Source: CAD feature listing. Evaluate the final solid. Frame: model axes, mm. A direction names the side the tool comes from. Round coordinates to 2 decimals unless told otherwise and drop trailing zeros. Loops run counter-clockwise (first coordinate to the right, second up) from the corner with the lowest first, then second, coordinate; pieces in that order, holes last. Notation, with made-up numbers: (-3, 16) -> (55, 16) arc R25 ccw to (55, 35) -> close; hole circle Ø7 at (-13.75, 45.25). An arc over 180 degrees is marked (long way). Write item = value, one per line.
from build123d import *

# Parameters (mm, degrees)
PAD_DEPTH      = 4
PAD_DEPTH_BACK = 4
SKETCH001_R    = 1.75
POCKET_DEPTH   = 5
CHAMFER_SIZE   = 1


with BuildPart() as part:
    # Sketch → Pad (new body, two sides)
    with BuildSketch(Plane.XY) as pad_sk:
        with BuildLine():
            ThreePointArc((-10.999985, 2.5), (-12.936486, 1.791293), (-13.95804, 0))
            Line((-13.95804, 0), (-16, 0))
            Line((-16, 0), (-16, 5))
            Line((-16, 5), (4, 5))
            Line((4, 5), (4, 0))
            Line((-4, 0), (4, 0))
            ThreePointArc((-4, 0), (-5.021548, 1.791287), (-6.958038, 2.5))
            Line((-10.999985, 2.5), (-6.958038, 2.5))
        make_face()
    extrude(amount=PAD_DEPTH)
    extrude(pad_sk.sketch, amount=-PAD_DEPTH_BACK)

    # Sketch001 → Pocket (cut)
    with BuildSketch(Plane.XZ):
        Circle(SKETCH001_R)
    extrude(amount=-POCKET_DEPTH, mode=Mode.SUBTRACT)

    # Chamfer
    chamfer_edges = [part.edges().sort_by_distance(p)[0] for p in [
        (-16, 2.5, 4),
        (-16, 2.5, -4),
        (4, 2.5, -4),
        (4, 2.5, 4),
    ]]
    chamfer(chamfer_edges, length=CHAMFER_SIZE)


solid = part.part
1. Line query: probe 1 along X at (y, z) = (0.3, 0.75); probe 2 along X at (y, z) = (0.6, 1); probe 3 along Z at (x, y) = (0, 1.4). Output: solid intervals per line, ascending. Write a range as from..to.
Evaluation:
probe_1 = -16..-13.89, -4.07..-1.58, 1.58..4
probe_2 = -16..-13.79, -4.17..-1.44, 1.44..4
probe_3 = -4..-1.75, 1.75..4
2. Section query A-A (z = 0). Return the cut outline in (x, y).
Evaluation:
outline = (-16, 0) -> (-13.96, 0) arc R3 cw to (-11, 2.5) -> (-6.96, 2.5) arc R3 cw to (-4, 0) -> (-1.75, 0) -> (-1.75, 5) -> (-16, 5) -> close; (1.75, 0) -> (4, 0) -> (4, 5) -> (1.75, 5) -> close
3. Section query B-B (y = 1.2). Return the cut outline in (x, z).
Evaluation:
outline = (-16, -3) -> (-15, -4) -> (-13.47, -4) -> (-13.47, 4) -> (-15, 4) -> (-16, 3) -> close; (-4.49, -4) -> (3, -4) -> (4, -3) -> (4, 3) -> (3, 4) -> (-4.49, 4) -> close; hole circle Ø3.5 at (0, 0)
4. Contact query for flat-ended pins moving along their axis: pin 1 Ø4.5 at (x, z) = (-10, -1) entering from -Y; pin 2 Ø4.5 at (x, z) = (0, 0) entering from +Y. Output: stop coordinate, or through.
Evaluation:
pin_1 = 2.23
pin_2 = 5
5. Set-up query: faces 5 (the face through (-12.914, 1.81, 0.056)), 6 (the face through (-6, 5, 0)). Return all of +Z, -Z, +X, -X, +Y, -Y with unobstructed straight access to the full face (end or side cutting, diameter ignored); none if empty.
Evaluation:
face_5 = +Z, -Z, -Y
face_6 = +Z, -Z, +X, -X, +Y
6. Section query D-D (y = 4.6). Return the cut outline in (x, z).
Evaluation:
outline = (-16, -3) -> (-15, -4) -> (3, -4) -> (4, -3) -> (4, 3) -> (3, 4) -> (-15, 4) -> (-16, 3) -> close; hole circle Ø3.5 at (0, 0)
7. Mould query, pull axis X, two halves, no side actions, for faces 1 (the face through (-16, 2, 0)), 2 (the face through (-9, 2.5, 0)), 3 (the face through (-6, 3, 4)), 4 (the face through (1.617, 2.465, -0.67)). Classes: released by +X, released by -X, zero draft, split by the parting line, or undercut.
Evaluation:
face_1 = released by -X
face_2 = undercut
face_3 = zero draft
face_4 = undercut
8. Section query C-C (x = 0). Return the cut outline in (y, z), then the cut area to 3 significant figures.
Evaluation:
outline = (0, -4) -> (5, -4) -> (5, -1.75) -> (0, -1.75) -> close; (0, 1.75) -> (5, 1.75) -> (5, 4) -> (0, 4) -> close
area = 22.5 mm²
